Autodesk Inventor part; units mm, degrees
ref_plane "YZ Plane" through (0, 0, 0) normal (1, 0, 0) x (0, 1, 0)
ref_plane "XZ Plane" through (0, 0, 0) normal (0, 1, 0) x (-1, 0, 0)
ref_plane "XY Plane" through (0, 0, 0) normal (0, 0, 1) x (1, 0, 0)
sketch "Sketch1" plane through (0, 0, 0) normal (0, 0, 1) x (1, 0, 0)
  line L0 (-5, 0) -> (5, 0)
  line L1 (5, 0) -> (5, 16)
  line L2 (5, 16) -> (-5, 16)
  line L3 (-5, 16) -> (-5, 0)
  point P0 (0, 0)
  dimension "d0" = 0
  dimension "d1" = 10
  dimension "d2" = 16
  dimension "d3" = 5
extrude "Extrusion1" add sketch "Sketch1" along normal mid plane 12
sketch "Sketch2" plane through (0, 0, 6) normal (0, 0, 1) x (1, 0, 0)
  line L0 (5, 16) -> (-5, 16)
  line L1 (-2, 16) -> (2, 16)
  line L2 (2, 16) -> (2, 5)
  line L3 (2, 5) -> (-2, 5)
  line L4 (-2, 5) -> (-2, 16)
  point P0 (0, 0)
  dimension "d6" = 11
  dimension "d7" = 4
  dimension "d8" = 2
extrude "Extrusion2" cut sketch "Sketch2" against normal through all
sketch "Sketch3" plane through (5, 0, 6) normal (1, 0, 0) x (0, 0, -1)
  circle A0 centre (6, 10) radius 3
  line L0 (0, 0) -> (12, 0)
  line L1 (12, 16) -> (0, 16)
  point P0 (6, 0)
  point P1 (6, 0)
  dimension "d11" = 6
  dimension "d12" = 6
hole "Hole1" at (5, 10, 0) direction (-1, 0, 0) diameter 6 end through all
fillet "Fillet1" radius 6 4 edges at (3.5, 16, 6) (3.5, 16, -6) (-3.5, 16, -6) (-3.5, 16, 6)
sketch "Sketch4" plane through (-5, 0, 6) normal (0, -1, 0) x (1, 0, 0)
  circle A0 centre (5, -6) radius 1.5
  dimension "d21" = 3
hole "Hole2" at (0, 0, 0) direction (0, 1, 0) diameter 2.459 depth 5
equation "\"d13\" = d12"
properties part number "Gripper_Link_Holder" material "Aluminum 6061"
For this review, take the finished solid that the model builds, in its own axes (mm). A direction names the side the tool comes from. Coordinates: 2 decimals unless noted, no trailing zeros. Loops run counter-clockwise (first coordinate to the right, second up) from the corner with the lowest first, then second, coordinate; pieces in that order, holes last. Notation, with made-up numbers: (48, 30.5) -> (91, 30.5) arc R9 cw to (91, 39.5) -> close; hole circle Ø10 at (14, 63.25). An arc over 180 degrees is marked (long way). Return JSON: item names as keys, results as strings. Group by question number.
(1) Consider section A-A, the plane x = 0. Give the boundary of the cut face in (y, z), plus the area to 3 significant figures.
(2) Consider section C-C, the plane z = -1.75. Give the boundary of the cut face in (x, y).
(3) To check wall thickness, follow L1, parallel to X at y = 3.9, z = 0; L2, parallel to X at y = 13, z = 2.75; L3, parallel to Z at x = 3.6, y = 10. State the ranges of each line that lie inside material, in increasing order.
(4) For pin 1 Ø1 at (x, z) = (0.5, -1) entering from +Y; pin 2 Ø5 at (y, z) = (9, 1.5) entering from -X, all flat-tipped, find the tip position at first contact; note any pin that passes through.
(5) Mouldability with a two-part tool opening along X and no side actions: class faces 3 (the cylindrical face through (-3.521, 14.289, -4.196)), 4 (the flat face through (2, 12, 3)), 5 (the flat face through (5, 6, 0)) as pulls with the +X half, pulls with the -X half, needs draft (parallel to the pull), parting line crosses it, or undercut.
(6) Tool access review of faces 1 (the flat face through (-0.1, 0, -1.4)), 2 (the flat face through (0, 5, 1.4)): name each direction out of +Z, -Z, +X, -X, +Y, -Y from which nothing blocks a thin tool from reaching the whole face with its end or side.
(7) Consider section B-B, the plane y = 6.5. Give the boundary of the cut face in (x, z).
Results below:
{
 "1": {"outline": "(0, -6) -> (5, -6) -> (5, -1.23) -> (0, -1.23) -> close; (0, 1.23) -> (5, 1.23) -> (5, 6) -> (0, 6) -> close", "area": "47.7 mm2"},
 "2": {"outline": "(-5, 0) -> (5, 0) -> (5, 7.56) -> (2, 7.56) -> (2, 5) -> (-2, 5) -> (-2, 7.56) -> (-5, 7.56) -> close; (-5, 12.44) -> (-2, 12.44) -> (-2, 15.74) -> (-5, 15.74) -> close; (2, 12.44) -> (5, 12.44) -> (5, 15.74) -> (2, 15.74) -> close"},
 "3": {"L1": "x = -5 to -1.23, 1.23 to 5", "L2": "x = -5 to -2, 2 to 5", "L3": "z = -6 to -3, 3 to 6"},
 "4": {"pin 1": "stops at y = 5", "pin 2": "stops at x = -5"},
 "5": {"face 3": "needs draft", "face 4": "undercut", "face 5": "pulls with the +X half"},
 "6": {"face 1": "+Z, -Z, +X, -X, -Y", "face 2": "+Z, -Z, +Y"},
 "7": {"outline": "(-5, -6) -> (-2, -6) -> (-2, 6) -> (-5, 6) -> close; (2, -6) -> (5, -6) -> (5, 6) -> (2, 6) -> close"}
}
